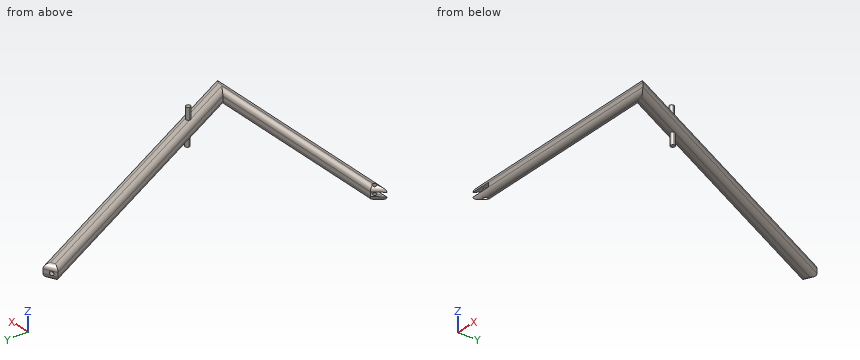
from build123d import *

# Parameters (mm, degrees)
BOSS_EXTRUDE1_DEPTH = 44.5
FILLET2_R           = 15
SKETCH2_R           = 7
CUT_EXTRUDE1_DEPTH  = 14
SKETCH3_R           = 7
CUT_EXTRUDE2_DEPTH  = 14
SKETCH4_R           = 7
CUT_EXTRUDE3_DEPTH  = 14
SKETCH5_R           = 7
CUT_EXTRUDE4_DEPTH  = 952.271625519
SKETCH6_W           = 14.5
SKETCH6_H           = 44.5
CUT_EXTRUDE5_DEPTH  = 936.632574619
BOSS_EXTRUDE3_DEPTH = 40
BOSS_EXTRUDE4_DEPTH = 40


with BuildPart() as part:
    # Sketch1 → Boss-Extrude1 (new body)
    with BuildSketch(Plane.XY):
        Polygon((-253.518736915, -141.579738071), (475.109189289, -141.579738071), (4.687860899, 822.926918688), (-35.308474161, 803.419402656), (409.63823983, -108.856554338), (-223.36176017, -108.856554338), align=None)
    extrude(amount=BOSS_EXTRUDE1_DEPTH)

    # Fillet2
    fillet2_edges = [part.edges().sort_by_distance(p)[0] for p in [
        (239.898525094, 340.673590309, 44.5),
        (-15.310306631, 813.173160672, 44.5),
        (187.164882834, 347.281424159, 44.5),
        (93.13823983, -108.856554338, 44.5),
        (-238.440248543, -125.218146204, 44.5),
        (93.13823983, -108.856554338, 0),
        (187.164882834, 347.281424159, 0),
        (-15.310306631, 813.173160672, 0),
        (239.898525094, 340.673590309, 0),
        (110.795226187, -141.579738071, 0),
        (-238.440248543, -125.218146204, 0),
        (110.795226187, -141.579738071, 44.5),
    ]]
    fillet(fillet2_edges, radius=FILLET2_R)

    # Sketch2 → Cut-Extrude1 (cut)
    with BuildSketch(Plane(origin=(-323.336767908, 662.938617367, 0), x_dir=(0.8987940462991654, 0.43837114678908073, 0), z_dir=(-0.43837114678908073, 0.8987940462991654, 0))):
        with Locations(Location((339.470196695, -21.913602874, 0), (0, 0, 180))):
            Circle(SKETCH2_R)
    extrude(amount=-CUT_EXTRUDE1_DEPTH, mode=Mode.SUBTRACT)

    # Sketch3 → Cut-Extrude2 (cut)
    with BuildSketch(Plane(origin=(-66.534083276, 61.316368798, 0), x_dir=(0, 0, 1), z_dir=(-0.735352443447444, 0.6776848706558778, 0))):
        with Locations(Location((22.366337019, -255.510068241, 0), (0, 0, 270))):
            Circle(SKETCH3_R)
    extrude(amount=-CUT_EXTRUDE2_DEPTH, mode=Mode.SUBTRACT)

    # Sketch4 → Cut-Extrude3 (cut)
    with BuildSketch(Plane(origin=(0, -141.579738071, 0), x_dir=(-1, 0, 0), z_dir=(0, -1, 0))):
        with Locations(Location((233.419507196, -21.201481555, 0), (0, 0, 117.634316404))):
            Circle(SKETCH4_R)
    extrude(amount=-CUT_EXTRUDE3_DEPTH, mode=Mode.SUBTRACT)

    # Sketch5 → Cut-Extrude4 (cut, through all)
    with BuildSketch(Plane.XY.offset(44.5)):
        with Locations(Location((-220.649115428, -125.427110978, 0), (0, 0, 350.522457382))):
            Circle(SKETCH5_R)
    extrude(amount=-CUT_EXTRUDE4_DEPTH, mode=Mode.SUBTRACT)

    # Sketch6 → Cut-Extrude5 (cut, through all)
    with BuildSketch(Plane(origin=(-66.534083276, 61.316368798, 0), x_dir=(0, 0, 1), z_dir=(-0.735352443447444, 0.6776848706558778, 0))):
        with Locations((22.25, -253.666818768)):
            Rectangle(SKETCH6_W, SKETCH6_H)
    extrude(amount=-CUT_EXTRUDE5_DEPTH, mode=Mode.SUBTRACT)

    # Sketch8 → Boss-Extrude3 (add)
    with BuildSketch(Plane.XY.offset(44.5)):
        with BuildLine():
            ThreePointArc((350.492241226, 46.628294304), (357.703100488, 46.229913436), (361.428471817, 52.416738718))
            ThreePointArc((361.428471817, 52.416738718), (354.659562876, 59.412923172), (347.443729839, 52.878668912))
            Line((347.443729839, 52.878668912), (350.492241226, 46.628294304))
        make_face()
        with BuildLine():
            Line((350.492241226, 46.628294304), (347.443729839, 52.878668912))
            ThreePointArc((347.443729839, 52.878668912), (348.136913493, 49.34814069), (350.492241226, 46.628294304))
        make_face()
    extrude(amount=BOSS_EXTRUDE3_DEPTH)

    # Sketch9 → Boss-Extrude4 (add)
    with BuildSketch(Plane(origin=(0, 0, 0), x_dir=(-1, 0, 0), z_dir=(0, 0, -1))):
        with BuildLine():
            ThreePointArc((-363.673348609, 52.680013675), (-356.190881193, 46.855723683), (-349.768761726, 53.831829624))
            ThreePointArc((-349.768761726, 53.831829624), (-353.191242582, 59.848585957), (-360.112006519, 59.981847043))
            Line((-360.112006519, 59.981847043), (-363.673348609, 52.680013675))
        make_face()
        with BuildLine():
            Line((-363.673348609, 52.680013675), (-360.112006519, 59.981847043))
            ThreePointArc((-360.112006519, 59.981847043), (-363.06032005, 56.900427651), (-363.673348609, 52.680013675))
        make_face()
    extrude(amount=BOSS_EXTRUDE4_DEPTH)


solid = part.part
Here's how the part is built. I have some questions about the finished solid (model axes, mm). Coordinates: 2 decimals unless noted, no trailing zeros. Order: outer loops, then holes, each group sorted by start corner. A loop starts at its lowest first (then second) coordinate and runs counter-clockwise, first axis right, second up. Notation, with made-up numbers: M 10,80 L 39,80 A17 cw 39,88 Z; hole C -21,47.5 d1. An arc over 180 degrees is marked long. Answer as CSV lines item,"result". Start each with the question number.
1. I need wall thicknesses on line 1 (Z direction, x = 92, y = 578); line 2 (Y direction, x = -93.5, z = 17); line 3 (X direction, y = 533.5, z = 5). Which ranges of each line are inside material? Lowest first, please. Write a range as [from, to].
2. I want a section at B-B, the plane z = 55.5. Write out the boundary of the cut face in (x, y).
3. For pin 1 (1.5 mm diameter, centred on x = 348.5, y = 48, fed in from -Z); pin 2 (3 mm diameter, centred on x = 361.5, y = 57.5, fed in from +Z); pin 3 (12 mm diameter, centred on y = 398, z = 29, fed in from -X); pin 4 (8.5 mm diameter, centred on x = -220.65, y = -125.43, fed in from -Z), each with a flat end and sliding along its axis, tell me the tip position at first contact or that it passes through.
4. I want a section at A-A, the plane x = -152. Write out the boundary of the cut face in (y, z).
Recorded:
1,line 1,"z = [0, 44.5]"
1,line 2,"y = [-141.58, -108.86]"
1,line 3,"x = [100.59, 141.6]"
2,outline,"C 354.43,52.42 d14"
3,pin 1,"stops at z = 0.01"
3,pin 2,"stops at z = 44.5"
3,pin 3,"stops at x = 159.5"
3,pin 4,"passes through"
4,outline,"M -141.58,15 A15 ccw -126.58,0 L -123.86,0 A15 ccw -108.86,15 L -108.86,29.5 A15 ccw -123.86,44.5 L -126.58,44.5 A15 ccw -141.58,29.5 Z"
